Input: part model. Units: mm. Frame: model coordinates. A direction names the side the tool comes from. Give positions to 0.01 mm unless a question says otherwise; leave off trailing zeros. Loops run counter-clockwise (first coordinate to the right, second up) from the corner with the lowest first, then second, coordinate; pieces in that order, holes last. Notation, with made-up numbers: M 29,28 L 79,28 A30 cw 79,58 Z; hole C 4,-22 d1. An arc over 180 degrees is marked long. Answer as a JSON object with one key per item and string values. Group by question number.
1) Section query D-D on x = -7.5. Return loops of the section in (y, z), plus the area to 3 significant figures.
2) Ray query, L1, parallel to Y at x = -8, z = 5; L2, parallel to X at y = -8, z = 2.5; L3, parallel to X at y = -13.5, z = 12.5. Return the intervals inside material, ascending.
3) Section query C-C on z = 11.5. Return loops of the section in (x, y).
4) First-contact query: P1, Ø2, axis at y = -10, z = 9, coming from the -X side; P2, Ø3.5, axis at x = 20.02, z = 4.28, coming from the +Y side; P3, Ø6, axis at y = -9.5, z = 7, coming from the +X side; P4, Ø3, axis at x = -15, y = -12, coming from the +Z side. Flat tips, straight axial feed; report the tip coordinate or a pass-through.
5) Section query A-A on x = 10. Return loops of the section in (y, z), plus the area to 3 significant figures.
6) Access query for faces 4 (the cylindrical face through (23.915, -15.338, 2.281)), 5 (the flat face through (13, -5.25, 6)), 6 (the flat face through (-13, -5.25, 6)). Directions: +Z, -Z, +X, -X, +Y, -Y. A direction counts if a zero-diameter tool reaches every point of the face in a straight line with its end or side. Return the directions, or none.
7) Draft query along X for faces 1 (the cylindrical face through (18.024, -15.412, 4.367)), 2 (the flat face through (6, -9, 8)), 3 (the cylindrical face through (-23.98, -2.59, 2.4)). Return one class per face: +X half, -X half, draft (parallel to the pull), parting line (faces both ways), or undercut.
8) Section query B-B on y = -4.5. Return loops of the section in (x, z), plus the area to 3 significant figures.
from build123d import *

# Parameters (mm, degrees)
F1_DEPTH = 18
F2_W     = 31.425511
F2_H     = 7.5
F3_DEPTH = 25
F4_R     = 2
F5_DEPTH = 25


with BuildPart() as f1:
    # F0 (on Front) → F1 (new body)
    with BuildSketch(Plane.XZ):
        with BuildLine():
            Line((-20, 0), (0, 0))
            Line((0, 0), (20, 0))
            ThreePointArc((20, 0), (23.947664, 2.33992), (23.789899, 6.926246))
            Line((23.789899, 6.926246), (6, 16.065147))
            Line((6, 16.065147), (-6, 16.065147))
            Line((-6, 16.065147), (-23.789899, 6.926246))
            ThreePointArc((-23.789899, 6.926246), (-23.947664, 2.33992), (-20, 0))
        make_face()
    extrude(amount=F1_DEPTH)

    # F2 (on face) → F3 (cut)
    with BuildSketch(Plane.XY.offset(16.065147)):
        with Locations((-21.712756, -9)):
            Rectangle(F2_W, F2_H)
        with Locations((21.712756, -9)):
            Rectangle(F2_W, F2_H)
    extrude(amount=-F3_DEPTH, mode=Mode.SUBTRACT)

    # F4 (on face) → F5 (cut)
    with BuildSketch(Plane.XZ.offset(18)):
        with Locations((-20, 4.5)):
            Circle(F4_R)
        with Locations((20.022377, 4.279106)):
            Circle(F4_R)
    extrude(amount=-F5_DEPTH, mode=Mode.SUBTRACT)


solid = f1.part
Output:
{
 "1": {"outline": "M -18,0 L -12.75,0 L -12.75,15.29 L -18,15.29 Z; M -5.25,0 L 0,0 L 0,15.29 L -5.25,15.29 Z", "area": "161 mm^2"},
 "2": {"L1": "y = -18 to -12.75, -5.25 to 0", "L2": "x = -6 to 6", "L3": "x = -12.94 to 12.94"},
 "3": {"outline": "M -14.89,-18 L 14.89,-18 L 14.89,-12.75 L 6,-12.75 L 6,-5.25 L 14.89,-5.25 L 14.89,0 L -14.89,0 L -14.89,-5.25 L -6,-5.25 L -6,-12.75 L -14.89,-12.75 Z"},
 "4": {"P1": "stops at x = -6", "P2": "passes through", "P3": "stops at x = 6", "P4": "stops at z = 12.11"},
 "5": {"outline": "M -18,0 L -12.75,0 L -12.75,14.01 L -18,14.01 Z; M -5.25,0 L 0,0 L 0,14.01 L -5.25,14.01 Z", "area": "147 mm^2"},
 "6": {"face 4": "+X, +Y, -Y", "face 5": "+Z, -Z, +X", "face 6": "+Z, -Z, -X"},
 "7": {"face 1": "undercut", "face 2": "+X half", "face 3": "-X half"},
 "8": {"outline": "M -23.79,6.93 A4.5 ccw -20,0 L 20,0 A4.5 ccw 23.79,6.93 L 6,16.07 L -6,16.07 Z; hole C -20,4.5 d4; hole C 20.02,4.28 d4", "area": "577 mm^2"}
}
